For this review, take the finished solid that the model builds, in its own axes (mm). Face numbers are marked on the shaded views. A direction names the side the tool comes from. Give positions to 0.01 mm unless a question says otherwise; leave off trailing zeros. Order: outer loops, then holes, each group sorted by start corner. A loop starts at its lowest first (then second) coordinate and runs counter-clockwise, first axis right, second up. Notation, with made-up numbers: M -16.75,-19 L 20.25,-19 A22 cw 20.25,18 Z; hole C -27.5,-34.75 d7. An arc over 180 degrees is marked long. Use CSV: the item, a comma, the result in double quotes. Start each with the question number.
(1) Tool access review of the marked faces 1 and 2: name each direction out of +Z, -Z, +X, -X, +Y, -Y from which nothing blocks a thin tool from reaching the whole face with its end or side.
(2) Wall thickness on L1, parallel to Y at x = 0.3, z = 2.6; L2, parallel to Y at x = -1.65, z = 0.45; L3, parallel to X at y = 11.5, z = 1.15: over which ranges is each line inside the solid? List them lowest first. Write a range as from..to.
(3) Consider section B-B (z = 0). Write out the cut boundary in (x, y).
(4) Consider section A-A (x = 0). Write out the cut boundary in (y, z), and give its area (3 significant figures).
(5) Consider section D-D (z = 1.1). Write out the cut boundary in (x, y).
(6) Consider section C-C (y = 9.25). Write out the cut boundary in (x, z).
(7) Clearance check with flat-ended pins moving along their axes: P1, Ø3, axis at y = 23, z = -1.5, coming from the +X side; P2, Ø1, axis at x = -2.5, y = 17, coming from the -Z side; P3, Ø0.6, axis at x = -0.5, y = 27, coming from the -Z side. State where each tip first meets the part, or that it passes through.
Solid Edge part; units mm, degrees
sketch "Sketch1" plane through (0, 0, 0) normal (0, -1, 0) x (1, 0, 0)
  circle A0 centre (0, 0) radius 1.5
extrude "Protrusion1" add sketch "Sketch1" against normal blind 25
sketch "Sketch2" plane through (0, 25, 0) normal (0, 1, 0) x (1, 0, 0)
  circle A0 centre (0, 0) radius 3
extrude "ExtrudedProtrusion_2" add sketch "Sketch2" along normal blind 2.52
sketch "Sketch3" plane through (0, 27.52, 0) normal (0, 1, 0) x (-1, 0, 0)
  line L0 (-2.9311, 0.6393) -> (2.9311, 0.6393)
  arc A0 (2.9311, 0.6393) -> (2.9311, -0.6393) centre (0, 0) cw
  line L1 (2.9311, -0.6393) -> (-2.9311, -0.6393)
  arc A1 (-2.9311, -0.6393) -> (-2.9311, 0.6393) centre (0, 0) cw
extrude "ExtrudedCutout_1" cut sketch "Sketch3" against normal blind 0.8
cosmetic_thread "Thread1"
properties material "Nylon, general purpose"
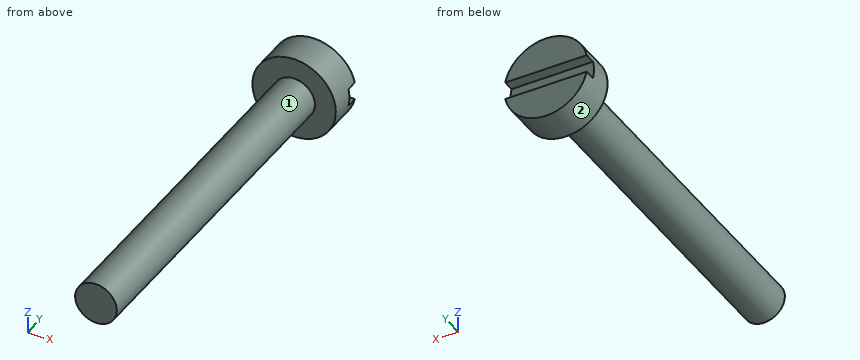
Check result:
1,face 1,"-Y"
1,face 2,"+Y, -Y"
2,L1,"y = 25..27.52"
2,L2,"y = 25..26.72"
2,L3,"x = -0.96..0.96"
3,outline,"M -3,25 L -1.5,25 L -1.5,0 L 1.5,0 L 1.5,25 L 3,25 L 3,26.72 L -3,26.72 Z"
4,outline,"M 0,-1.5 L 25,-1.5 L 25,-3 L 27.52,-3 L 27.52,-0.64 L 26.72,-0.64 L 26.72,0.64 L 27.52,0.64 L 27.52,3 L 25,3 L 25,1.5 L 0,1.5 Z"
4,area,"89.1 mm^2"
5,outline,"M -2.79,25 L -1.02,25 L -1.02,0 L 1.02,0 L 1.02,25 L 2.79,25 L 2.79,27.52 L -2.79,27.52 Z"
6,outline,"C 0,0 d3"
7,P1,"stops at x = 1.5"
7,P2,"passes through"
7,P3,"stops at z = -2.99"
